```python
from build123d import *

# Parameters (mm, degrees)
SKETCH2_R          = 2.15
CUT_EXTRUDE1_DEPTH = 5
CIRPATTERN1_COUNT  = 4


with BuildPart() as part:
    # Sketch1 → Revolve4 (revolve)
    with BuildSketch(Plane(origin=(0, 0, 0), x_dir=(0, 0, -1), z_dir=(1, 0, 0))):
        Polygon((8, 0), (8, -10), (16, -10), (16, -14), (5, -14), (5, 0), align=None)
    revolve(axis=Axis((0, 0, 0), (0, -1, 0)))

    # Sketch2 → Cut-Extrude1 (cut, through all)
    with BuildSketch(Plane(origin=(0, -10, 0), x_dir=(1, 0, 0), z_dir=(0, 1, 0))):
        with Locations((-12, 0)):
            Circle(SKETCH2_R)
    cut_extrude1 = extrude(amount=-CUT_EXTRUDE1_DEPTH, mode=Mode.SUBTRACT)

    # CirPattern1: Cut-Extrude1 ×4 about axis
    cirpattern1_axis = Axis((0, 0, 0), (0, 1, 0))
    for i in range(1, CIRPATTERN1_COUNT):
        add(cut_extrude1.rotate(cirpattern1_axis, i * 360 / CIRPATTERN1_COUNT), mode=Mode.SUBTRACT)


solid = part.part
```
Source: CAD feature listing. Evaluate the final solid. Frame: model axes, mm. A direction names the side the tool comes from. Round coordinates to 2 decimals unless told otherwise and drop trailing zeros. Loops run counter-clockwise (first coordinate to the right, second up) from the corner with the lowest first, then second, coordinate; pieces in that order, holes last. Notation, with made-up numbers: M 64.5,-35 L 105.5,-35 A26 cw 105.5,-6 Z; hole C 35,35 d5. An arc over 180 degrees is marked long. Use a Markdown table: item, result. Add a question column.
1. Contact query for flat-ended pins moving along their axis: P1, Ø8, axis at x = 1, y = -4.5, coming from the -Z side; P2, Ø5.5, axis at x = 0, z = -12, coming from the +Y side; P3, Ø3, axis at y = -8, z = 6, coming from the +X side; P4, Ø4, axis at x = 12, z = 0, coming from the -Y side. Output: stop coordinate, or through.
2. Section query B-B on x = 0. Return the cut outline in (y, z).
3. Section query A-A on z = 0. Return the cut outline in (x, y), then the cut area to 3 significant figures.
4. Reachability of faces 4 (the cylindrical face through (-7.81, -5.07, 1.73)), 5 (the cylindrical face through (-4.88, -6.9, 1.08)) from +Z, -Z, +X, -X, +Y, -Y: full face, straight path, thin tool, end or side. Return the list, or none.
5. Section query D-D on y = -1.5. Return the cut outline in (x, z).
6. Section query C-C on z = 11.5. Return the cut outline in (x, y), then the cut area to 3 significant figures.
7. Mould query, pull axis Z, two halves, no side actions, for faces 1 (the cylindrical face through (-9.95, -11.97, -0.65)), 2 (the cylindrical face through (-15.62, -12.03, 3.47)), 3 (the flat face through (3.8, -10, -7.3)). Classes: pulls with the +Z half, pulls with the -Z half, needs draft (parallel to the pull), parting line crosses it, or undercut.
8. Line query: line 1 (X direction, y = -8, z = 0); line 2 (Z direction, x = -1, y = -13.25); line 3 (Y direction, x = -6, z = 11). Output: solid intervals per line, ascending.
Reported:
| question | item | result |
|---|---|---|
| 1 | P1 | stops at z = -8 |
| 1 | P2 | stops at y = -10 |
| 1 | P3 | stops at x = 6.61 |
| 1 | P4 | passes through |
| 2 | outline | M -14,-16 L -10,-16 L -10,-14.15 L -14,-14.15 Z; M -14,-9.85 L -10,-9.85 L -10,-8 L 0,-8 L 0,-5 L -14,-5 Z; M -14,5 L 0,5 L 0,8 L -10,8 L -10,9.85 L -14,9.85 Z; M -14,14.15 L -10,14.15 L -10,16 L -14,16 Z |
| 3 | outline | M -16,-14 L -14.15,-14 L -14.15,-10 L -16,-10 Z; M -9.85,-14 L -5,-14 L -5,0 L -8,0 L -8,-10 L -9.85,-10 Z; M 5,-14 L 9.85,-14 L 9.85,-10 L 8,-10 L 8,0 L 5,0 Z; M 14.15,-14 L 16,-14 L 16,-10 L 14.15,-10 Z |
| 3 | area | 114 mm² |
| 4 | face 4 | +Y |
| 4 | face 5 | +Y, -Y |
| 5 | outline | C 0,0 d16; hole C 0,0 d10 |
| 6 | outline | M -11.12,-14 L -2.09,-14 L -2.09,-10 L -11.12,-10 Z; M 2.09,-14 L 11.12,-14 L 11.12,-10 L 2.09,-10 Z |
| 6 | area | 72.3 mm² |
| 7 | face 1 | undercut |
| 7 | face 2 | parting line crosses it |
| 7 | face 3 | needs draft |
| 8 | line 1 | x = -8 to -5, 5 to 8 |
| 8 | line 2 | z = -15.97 to -13.9, -10.1 to -4.9, 4.9 to 10.1, 13.9 to 15.97 |
| 8 | line 3 | y = -14 to -10 |
